Design review of the part built by this model. Coordinates are the model's own, in mm. Give positions to 0.01 mm unless a question says otherwise; leave off trailing zeros. Order: outer loops, then holes, each group sorted by start corner. A loop starts at its lowest first (then second) coordinate and runs counter-clockwise, first axis right, second up. Notation, with made-up numbers: (49.5, 85) -> (98.5, 85) arc R21 ccw to (98.5, 112) -> close; hole circle Ø10 at (56.25, 1). An arc over 180 degrees is marked (long way). One line per item, written item: value.
Solid Edge part; units mm, degrees
sketch "Sketch1" plane through (0, 0, 0) normal (0, 0, 1) x (1, 0, 0)
  circle A0 centre (0, 0) radius 15.5
  circle A1 centre (0, 0) radius 27.5
extrude "Protrusion1" add sketch "Sketch1" along normal blind 3
hole "Hole_1" at (-21.5, 0, 3) direction (0, 0, -1) diameter 3.5 end up to next
hole "Hole1" at (0, -21.5, 3) direction (0, 0, -1) diameter 3.5 end up to next
hole "Hole2" at (21.5, 0, 3) direction (0, 0, -1) diameter 3.5 end up to next
hole "Hole3" at (0, 21.5, 3) direction (0, 0, -1) diameter 3.5 end up to next
properties material "Aluminum, 6061-T6"
Item 1: Add section C-C on z = 2.55. Give the boundary of the cut face in (x, y), plus the area to 3 significant figures.
Returned:
outline: circle Ø55 at (0, 0); hole circle Ø3.5 at (-21.5, 0); hole circle Ø31 at (0, 0); hole circle Ø3.5 at (0, -21.5); hole circle Ø3.5 at (0, 21.5); hole circle Ø3.5 at (21.5, 0)
area: 1,580 mm²
Item 2: Clearance check with flat-ended pins moving along their axes: P1, Ø1.5, axis at x = -20, z = 2.5, coming from the +Y side; P2, Ø1.5, axis at x = -18, z = 2, coming from the -Y side; P3, Ø1.5, axis at x = 8.5, z = 2, coming from the -Y side. State where each tip first meets the part, or that it passes through.
Returned:
P1: y = 19.64
P2: y = -21.42
P3: y = -26.39
Item 3: Add section A-A on x = 0. Give the boundary of the cut face in (y, z), plus the area to 3 significant figures.
Returned:
outline: (-27.5, 0) -> (-23.25, 0) -> (-23.25, 3) -> (-27.5, 3) -> close; (-19.75, 0) -> (-15.5, 0) -> (-15.5, 3) -> (-19.75, 3) -> close; (15.5, 0) -> (19.75, 0) -> (19.75, 3) -> (15.5, 3) -> close; (23.25, 0) -> (27.5, 0) -> (27.5, 3) -> (23.25, 3) -> close
area: 51.0 mm²
Item 4: To check wall thickness, follow line 1 along Y through (x, z) = (0, 1.3); line 2 along Y through (x, z) = (1.5, 2.8); line 3 along X through (y, z) = (8, 0.9). State the ranges of each line that lie inside material, in increasing order. Write a range as from..to.
Returned:
line 1: -27.5..-23.25, -19.75..-15.5, 15.5..19.75, 23.25..27.5
line 2: -27.46..-22.4, -20.6..-15.43, 15.43..20.6, 22.4..27.46
line 3: -26.31..-13.28, 13.28..26.31
Item 5: Draft analysis for pull direction Y (two halves, no side actions). For faces 1 (the cylindrical face through (0.08, 23.25, 1.52)), 2 (the flat face through (12, -12, 0)), 3 (the cylindrical face through (-5.961, 26.846, 1.479)), state which applies: pulls with the +Y half, pulls with the -Y half, needs draft (parallel to the pull), parting line crosses it, or undercut.
Returned:
face 1: undercut
face 2: needs draft
face 3: parting line crosses it
Item 6: Add section D-D on y = -21.5. Give the boundary of the cut face in (x, z).
Returned:
outline: (-17.15, 0) -> (-1.75, 0) -> (-1.75, 3) -> (-17.15, 3) -> close; (1.75, 0) -> (17.15, 0) -> (17.15, 3) -> (1.75, 3) -> close
